The model under review builds one solid part; all positions refer to its coordinate system, in mm. A direction names the side the tool comes from. Round coordinates to 2 decimals unless told otherwise and drop trailing zeros. Loops run counter-clockwise (first coordinate to the right, second up) from the corner with the lowest first, then second, coordinate; pieces in that order, holes last. Notation, with made-up numbers: M -15.75,19.5 L 23.25,19.5 A22 cw 23.25,48.5 Z; hole C 84,76.5 d9. An arc over 180 degrees is marked long. Answer in a Markdown table with one row per item. Add a question column.
Solid Edge part; units mm, degrees
sketch "Sketch1" plane through (0, 0, 0) normal (0, 0, 1) x (1, 0, 0)
  line L0 (-78.7684, 102.3579) -> (-70.7684, 102.3579)
  line L1 (-70.7684, 102.3579) -> (-70.7684, 30.3579)
  line L2 (-70.7684, 30.3579) -> (38.2316, 30.3579)
  line L3 (38.2316, 30.3579) -> (38.2316, 102.3579)
  line L4 (38.2316, 102.3579) -> (46.2316, 102.3579)
  line L5 (46.2316, 102.3579) -> (46.2316, 22.3579)
  line L6 (46.2316, 22.3579) -> (-78.7684, 22.3579)
  line L7 (-78.7684, 22.3579) -> (-78.7684, 102.3579)
  dimension "D1" = 78.7684
extrude "Protrusion1" add sketch "Sketch1" along normal blind 195
hole "Hole_1" at (46.2316, 43.3579, 120) direction (-1, 0, 0) diameter 6.5 end up to next
hole "Hole1" at (46.2316, 43.3579, 70) direction (-1, 0, 0) diameter 6.5 end up to next
hole "Hole2" at (46.2316, 43.3579, 170) direction (-1, 0, 0) diameter 6.5 end up to next
sketch "Sketch2" plane through (-16.2684, 22.3579, 75) normal (0, -1, 0) x (1, 0, 0)
  circle A0 centre (0, 29.5) radius 5
extrude "Cutout1" cut sketch "Sketch2" against normal through all
sketch "Sketch3" plane through (-16.2684, 22.3579, 75) normal (0, -1, 0) x (1, 0, 0)
  circle A0 centre (0, 29.5) radius 12.5
extrude "ExtrudedCutout_2" cut sketch "Sketch3" against normal blind 1
hole "Hole_6" at (-78.7684, 43.7635, 19.5944) direction (1, 0, 0) diameter 6.5 end up to next
hole "Hole3" at (-78.7684, 43.7635, 80.4056) direction (1, 0, 0) diameter 6.5 end up to next
properties material "Aluminum, 6061-T6"
1. Mouldability with a two-part tool opening along Z and no side actions: class faces 1 (the flat face through (-21, 30, 0)), 2 (the flat face through (-75, 102.358, 96)), 3 (the cylindrical face through (-74.824, 41.786, 17.015)) as released by +Z, released by -Z, zero draft, split by the parting line, or undercut.
2. Take a section at A-A, the plane z = 70. State the section outline as (x, y) points, and give its area (3 significant figures).
3. For pin 1 Ø22.5 at (x, z) = (-16.27, 104.5) entering from -Y; pin 2 Ø8 at (x, z) = (-37, 61) entering from +Y; pin 3 Ø6 at (y, z) = (43.36, 170) entering from +X, all flat-tipped, find the tip position at first contact; note any pin that passes through.
4. Take a section at C-C, the plane z = 46. State the section outline as (x, y) points, and give its area (3 significant figures).
5. Machinability: for faces 4 (the cylindrical face through (-74.824, 41.786, 77.827)), 5 (the cylindrical face through (42.288, 40.475, 118.5)), 6 (the flat face through (-70.768, 67, 96)), 7 (the flat face through (-16, 23.358, 99)), which of the approach directions +Z, -Z, +X, -X, +Y, -Y give a long, thin tool a straight path to every point of the face, cutting with its end or side? Answer none if there is none.
6. Take a section at B-B, the plane y = 76.5. State the section outline as (x, z) points.
7. To check wall thickness, follow probe 1 along X at (y, z) = (66, 185.5); probe 2 along Y at (x, z) = (41, 120); probe 3 along Y at (x, z) = (-23, 87.5). State the ranges of each line that lie inside material, in increasing order.
8. Take a section at D-D, the plane z = 104.5. State the section outline as (x, y) points, and give its area (3 significant figures).
Check sheet entries:
| question | item | result |
|---|---|---|
| 1 | face 1 | released by -Z |
| 1 | face 2 | zero draft |
| 1 | face 3 | undercut |
| 2 | outline | M -78.77,22.36 L 46.23,22.36 L 46.23,40.11 L 38.23,40.11 L 38.23,30.36 L -70.77,30.36 L -70.77,102.36 L -78.77,102.36 Z; M 38.23,46.61 L 46.23,46.61 L 46.23,102.36 L 38.23,102.36 Z |
| 2 | area | 2,100 mm^2 |
| 3 | pin 1 | stops at y = 23.36 |
| 3 | pin 2 | stops at y = 30.36 |
| 3 | pin 3 | stops at x = -70.77 |
| 4 | outline | M -78.77,22.36 L 46.23,22.36 L 46.23,102.36 L 38.23,102.36 L 38.23,30.36 L -70.77,30.36 L -70.77,102.36 L -78.77,102.36 Z |
| 4 | area | 2,150 mm^2 |
| 5 | face 4 | -X |
| 5 | face 5 | +X |
| 5 | face 6 | +Z, -Z, +Y |
| 5 | face 7 | -Y |
| 6 | outline | M -78.77,0 L -70.77,0 L -70.77,195 L -78.77,195 Z; M 38.23,0 L 46.23,0 L 46.23,195 L 38.23,195 Z |
| 7 | probe 1 | x = -78.77 to -70.77, 38.23 to 46.23 |
| 7 | probe 2 | y = 22.36 to 40.11, 46.61 to 102.36 |
| 7 | probe 3 | y = 22.36 to 30.36 |
| 8 | outline | M -78.77,22.36 L -28.77,22.36 L -28.77,23.36 L -21.27,23.36 L -21.27,30.36 L -70.77,30.36 L -70.77,102.36 L -78.77,102.36 Z; M -11.27,23.36 L -3.77,23.36 L -3.77,22.36 L 46.23,22.36 L 46.23,102.36 L 38.23,102.36 L 38.23,30.36 L -11.27,30.36 Z |
| 8 | area | 2,060 mm^2 |
